Geometry: final body of the model. Coordinates: model frame, mm. Face numbers are marked on the shaded views. A direction names the side the tool comes from. Round coordinates to 2 decimals unless told otherwise and drop trailing zeros. Order: outer loops, then holes, each group sorted by start corner. A loop starts at its lowest first (then second) coordinate and runs counter-clockwise, first axis right, second up. Notation, with made-up numbers: (-10.5, 64.25) - (-4.5, 64.25) arc R16 ccw to (-4.5, 71.25) - close; hole circle Ø6 at (-28, 19). An arc over 180 degrees is marked (long way). Put each result on its own line as item: value. Start each with the question number.
(1) Section D-D (x = 3.5). Output: boundary loops of the cut face in (y, z) (3 decimals), and give its area (3 significant figures).
(2) Section A-A (z = 5.5). Count the separate pieces of the cut face and the enclosed holes in it, and give its area (3 significant figures).
(3) Pin query (flat end, axial travel): P1, Ø1.5, axis at y = -4.5, z = 14, coming from the +X side; P2, Ø4, axis at x = 14, y = -4, coming from the +Z side; P3, Ø10, axis at x = 1.5, z = 15, coming from the +Y side. Return the tip coordinate at first contact, or that it passes through.
(4) Section C-C (x = 14). Output: boundary loops of the cut face in (y, z).
(5) Material intervals for L1, parallel to Y at x = 0, z = 4.6; L2, parallel to Y at x = -12.7, z = 5 (3 decimals); L3, parallel to Z at x = -9, y = -16.5, sorted ascending. Write a range as [from, to].
(6) Pull-direction query (X, two-part tool) for the marked faces 1, 2, 3 and 4; classes: released by +X, released by -X, zero draft, split by the parting line, or undercut.
(7) Access query for the marked faces 5 and 6. Directions: +Z, -Z, +X, -X, +Y, -Y. A direction counts if a zero-diameter tool reaches every point of the face in a straight line with its end or side. Return the directions, or none.
from build123d import *

# Parameters (mm, degrees)
F0_W     = 38.1
F0_H     = 38.1
F1_DEPTH = 6.35
F3_D     = 6.35
F4_R     = 6.35
F5_R     = 8.5725
F6_DEPTH = 12.7
F7_R     = 11.7475
F7_R_2   = 8.5725
F8_DEPTH = 3.175


with BuildPart() as f1:
    # F0 (on Top) → F1 (new body)
    with BuildSketch(Plane.XY):
        Rectangle(F0_W, F0_H)
    extrude(amount=F1_DEPTH)

    # F3 (through all)
    with Locations(Plane.XY.offset(6.35)):
        with Locations((-12.7, 12.7), (-12.7, -12.7), (12.7, -12.7), (12.7, 12.7)):
            Hole(F3_D / 2)

    # F4
    f4_edges = [f1.edges().sort_by_distance(p)[0] for p in [
        (-19.05, -19.05, 3.175),
        (19.05, -19.05, 3.175),
        (19.05, 19.05, 3.175),
        (-19.05, 19.05, 3.175),
    ]]
    fillet(f4_edges, radius=F4_R)

    # F5 (on face) → F6 (join)
    with BuildSketch(Plane.XY.offset(6.35)):
        Circle(F5_R)
    extrude(amount=F6_DEPTH)

    # F7 (on face) → F8 (cut)
    with BuildSketch(Plane.XY.offset(6.35)):
        Circle(F7_R)
        Circle(F7_R_2, mode=Mode.SUBTRACT)
    extrude(amount=-F8_DEPTH, mode=Mode.SUBTRACT)


solid = f1.part
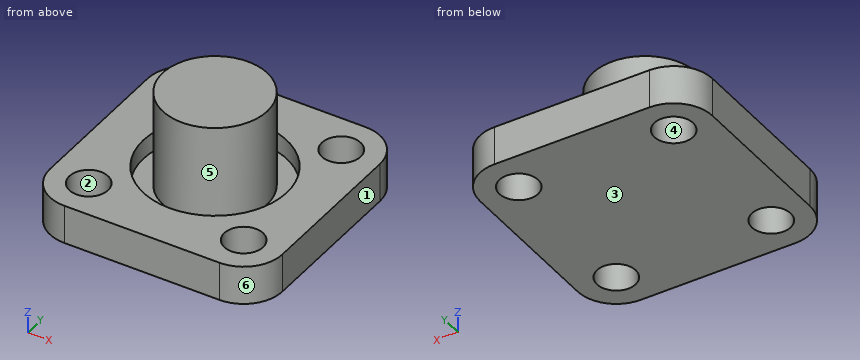
Checks:
1. outline: (-19.05, 0) - (19.05, 0) - (19.05, 6.35) - (11.214, 6.35) - (11.214, 3.175) - (7.825, 3.175) - (7.825, 19.05) - (-7.825, 19.05) - (-7.825, 3.175) - (-11.214, 3.175) - (-11.214, 6.35) - (-19.05, 6.35) - close
1. area: 419 mm²
2. separate pieces: 2
2. enclosed holes: 5
2. area: 1,090 mm²
3. P1: stops at x = 7.71
3. P2: stops at z = 6.35
3. P3: stops at y = 8.57
4. outline: (-18.92, 0) - (-15.6, 0) - (-15.6, 6.35) - (-18.92, 6.35) - close; (-9.8, 0) - (9.8, 0) - (9.8, 6.35) - (-9.8, 6.35) - close; (15.6, 0) - (18.92, 0) - (18.92, 6.35) - (15.6, 6.35) - close
5. L1: y = [-19.05, -11.75], [-8.57, 8.57], [11.75, 19.05]
5. L2: y = [-19.05, -15.875], [-9.525, 9.525], [15.875, 19.05]
5. L3: z = [0, 6.35]
6. face 1: released by +X
6. face 2: undercut
6. face 3: zero draft
6. face 4: undercut
7. face 5: +Z
7. face 6: +Z, -Z, +X, -Y
